The drawing under review shows one solid part. Ordinate dimensions are in mm from its lowest x, y, z. A direction names the side the tool comes from. Give positions to 0.01 mm unless a question says otherwise; leave off trailing zeros. Order: outer loops, then holes, each group sorted by start corner. A loop starts at its lowest first (then second) coordinate and runs counter-clockwise, first axis right, second up. Notation, with made-up numbers: (54.25, -7.75) -> (99.25, -7.75) arc R30 cw to (99.25, 23.25) -> close; hole circle Ø9 at (42.25, 17). An arc over 180 degrees is marked (long way). Return JSON: item names as keys, results as strings. Group by question number.
1) Add section D-D (y = 38.5). Give the boundary of the cut face in (x, z), then the cut area to 3 significant figures.
2) Add section A-A (z = 26.5). Give the boundary of the cut face in (x, y), then the cut area to 3 significant figures.
3) Add section C-C (x = 22). Give the boundary of the cut face in (y, z), then the cut area to 3 significant figures.
4) Add section B-B (y = 10). Give the boundary of the cut face in (x, z).
5) For the marked faces 1, 2 and 3, list the 3-axis set-ups (+Z, -Z, +X, -X, +Y, -Y) from which the entire face can be reached by the end or side of a thin tool; tool diameter is ignored.
6) The part is to be moulded in two halves that separate along Z. For the marked faces 4, 5 and 6, say which applies: released by +Z, released by -Z, zero draft, split by the parting line, or undercut.
7) To check wall thickness, follow line 1 along Z through (x, y) = (33, 10); line 2 along Z through (x, y) = (48.5, 33.5); line 3 along X through (y, z) = (17, 217). State the ranges of each line that lie inside material, in increasing order.
8) Insertion check: P1, Ø5.5, axis at y = 56, z = 2.5, coming from the -X side; P2, Ø1.6, axis at x = 36, z = 210.5, coming from the +Y side; P3, Ø5.5, axis at y = 56, z = 2, coming from the +X side. Each pin has a flat end and moves straight along its axis. Give the tip position at first contact, or say it passes through.
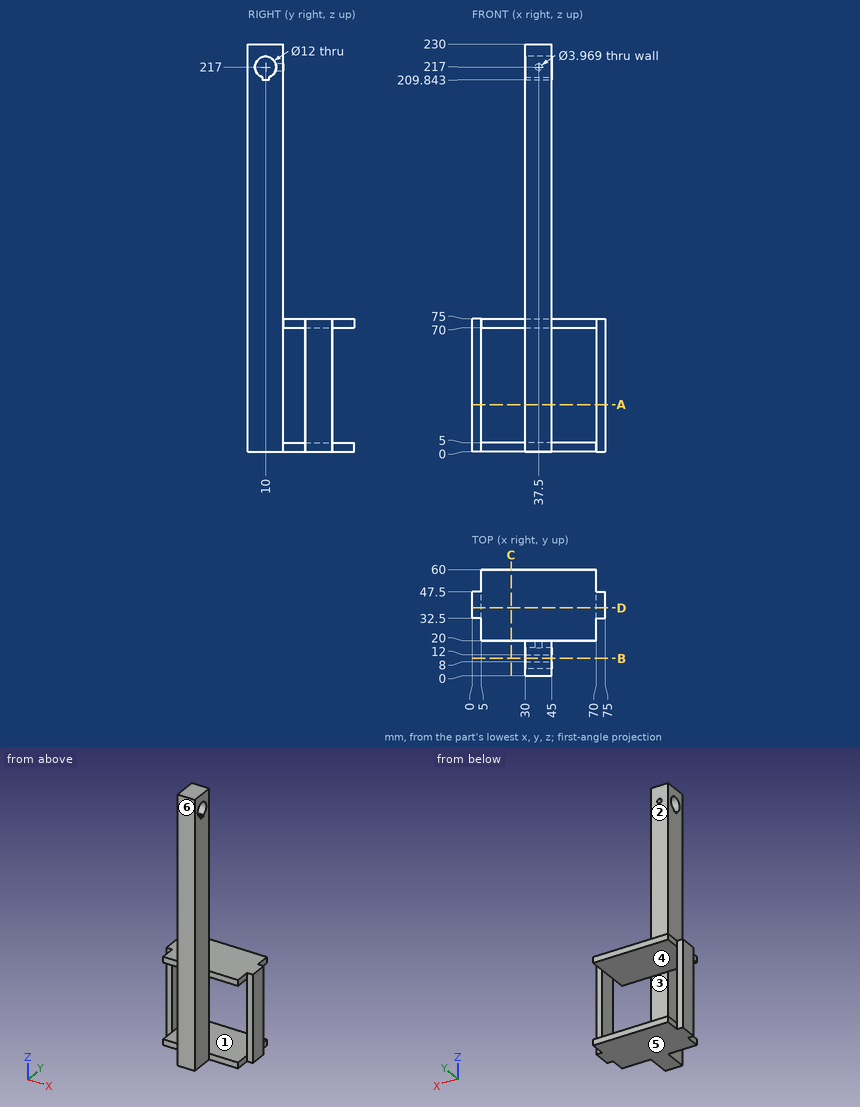
Evaluation:
{
 "1": {"outline": "(0, 0) -> (75, 0) -> (75, 75) -> (0, 75) -> close; hole (5, 5) -> (70, 5) -> (70, 70) -> (5, 70) -> close", "area": "1,400 mm^2"},
 "2": {"outline": "(0, 32.5) -> (5, 32.5) -> (5, 47.5) -> (0, 47.5) -> close; (30, 0) -> (45, 0) -> (45, 20) -> (30, 20) -> close; (70, 32.5) -> (75, 32.5) -> (75, 47.5) -> (70, 47.5) -> close", "area": "450 mm^2"},
 "3": {"outline": "(20, 0) -> (60, 0) -> (60, 5) -> (20, 5) -> close; (20, 70) -> (60, 70) -> (60, 75) -> (20, 75) -> close", "area": "400 mm^2"},
 "4": {"outline": "(30, 0) -> (45, 0) -> (45, 209.84) -> (30, 209.84) -> close; (30, 223) -> (45, 223) -> (45, 230) -> (30, 230) -> close"},
 "5": {"face 1": "+Y", "face 2": "+Z, +X, -X, +Y", "face 3": "+X, -X, +Y"},
 "6": {"face 4": "undercut", "face 5": "released by -Z", "face 6": "zero draft"},
 "7": {"line 1": "0 to 209.84, 223 to 230", "line 2": "0 to 5, 70 to 75", "line 3": "30 to 35.52, 39.48 to 45"},
 "8": {"P1": "x = 5", "P2": "y = 20", "P3": "x = 70"}
}
